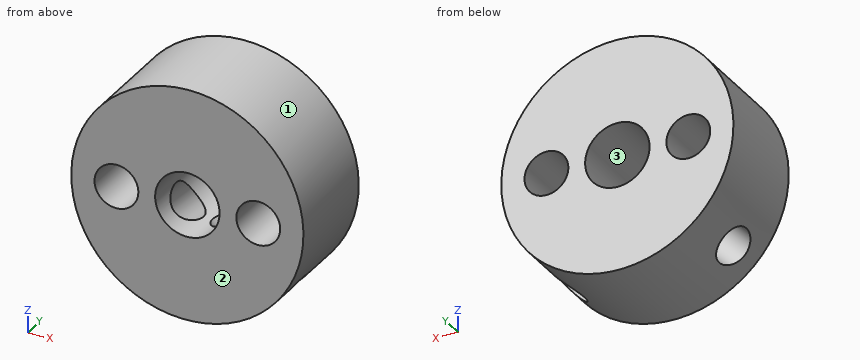
from build123d import *

# Parameters (mm, degrees)
SKETCH1_R           = 9
SKETCH1_R_2         = 2.5
SKETCH1_R_3         = 1.7
BOSS_EXTRUDE1_DEPTH = 8
SKETCH2_R           = 1.5
CUT_EXTRUDE1_DEPTH  = 16.033296378


with BuildPart() as part:
    # Sketch1 → Boss-Extrude1 (new body)
    with BuildSketch(Plane(origin=(0, 0, 0), x_dir=(1, 0, 0), z_dir=(0, 1, 0))):
        with Locations(Location((0, 0, 0), (0, 0, 270))):
            Circle(SKETCH1_R)
        with Locations(Location((0, 0, 0), (0, 0, 270))):
            Circle(SKETCH1_R_2, mode=Mode.SUBTRACT)
        with Locations(Location((5.5, 0, 0), (0, 0, 270))):
            Circle(SKETCH1_R_3, mode=Mode.SUBTRACT)
        with Locations(Location((-5.5, 0, 0), (0, 0, 90))):
            Circle(SKETCH1_R_3, mode=Mode.SUBTRACT)
    extrude(amount=BOSS_EXTRUDE1_DEPTH)

    # Sketch2 → Cut-Extrude1 (cut, through all)
    with BuildSketch(Plane(origin=(0, 0, 0), x_dir=(0, -1, 0), z_dir=(-0.7071067811865488, 0, 0.7071067811865464))):
        with Locations(Location((-3, 0, 0), (0, 0, 90))):
            Circle(SKETCH2_R)
    cut_extrude1 = extrude(amount=-CUT_EXTRUDE1_DEPTH, mode=Mode.SUBTRACT)

    # Mirror1: Cut-Extrude1 across plane
    add(cut_extrude1.mirror(Plane(origin=(0, 0, 0), x_dir=(0, 0, 1), z_dir=(1, 0, 0))), mode=Mode.SUBTRACT)


solid = part.part
Can you work these out from the model? Positions are in its coordinate system, mm. Face numbers are marked on the shaded views. Coordinates: 2 decimals unless noted, no trailing zeros. Order: outer loops, then holes, each group sorted by start corner. A loop starts at its lowest first (then second) coordinate and runs counter-clockwise, first axis right, second up. Notation, with made-up numbers: M 36.5,56.25 L 81.5,56.25 A33 ccw 81.5,91.25 Z; hole C 22.25,21.25 d4. An arc over 180 degrees is marked long. Write item = value, one per line.
(1) Suppose I cut it at A-A on x = 0. Please give me the cut outline in (y, z), plus the area to 3 significant figures.
Results are:
outline = M 0,-9 L 8,-9 L 8,-2.5 L 0,-2.5 Z; M 0,2.5 L 8,2.5 L 8,9 L 0,9 Z
area = 104 mm2
(2) For pin 1 Ø1 at (y, z) = (1, 5) entering from +X; pin 2 Ø4 at (x, z) = (0, 0) entering from -Y; pin 3 Ø2 at (x, y) = (3.5, 7) entering from -Z; pin 4 Ø2 at (y, z) = (4.5, -1.5) entering from +X, each with a flat end and sliding along its axis, tell me the tip position at first contact or that it passes through.
Results are:
pin_1 = 7.79
pin_2 = through
pin_3 = -8.65
pin_4 = 8.99
(3) Suppose I cut it at D-D on y = 5. Please give me the cut outline in (x, z), plus the area to 3 significant figures.
Results are:
outline = C 0,0 d18; hole C -5.5,0 d3.4; hole C 0,0 d5; hole C 5.5,0 d3.4
area = 217 mm2
(4) If we mould it in two halves opening along Z, with no side actions, what happens to the marked faces 1, 2 and 3? For each: pulls with the +Z half, pulls with the -Z half, needs draft (parallel to the pull), parting line crosses it, or undercut.
Results are:
face_1 = parting line crosses it
face_2 = needs draft
face_3 = undercut
(5) Suppose I cut it at C-C on z = 0. Please give me the cut outline in (x, y), plus the area to 3 significant figures.
Results are:
outline = M -9,0 L -7.2,0 L -7.2,8 L -9,8 Z; M -3.8,0 L -2.5,0 L -2.5,8 L -3.8,8 Z; M 2.5,0 L 3.8,0 L 3.8,8 L 2.5,8 Z; M 7.2,0 L 9,0 L 9,8 L 7.2,8 Z
area = 49.6 mm2
(6) I need wall thicknesses on line 1 along X through (y, z) = (5, 0); line 2 along Z through (x, y) = (4, 3.75); line 3 along Z through (x, y) = (-6, 6). Which ranges of each line are inside material? Lowest first, please. Write a range as [from, to].
Results are:
line_1 = [-9, -7.2], [-3.8, -2.5], [2.5, 3.8], [7.2, 9]
line_2 = [-8.06, -5.84], [-2.16, -0.8], [0.8, 8.06]
line_3 = [-6.71, -1.62], [1.62, 6.71]
(7) Suppose I cut it at B-B on y = 4. Please give me the cut outline in (x, z).
Results are:
outline = M -7.11,-5.52 L -2.37,-0.79 A2.5 cw long 2.37,-0.79 L 7.11,-5.52 A9 ccw long Z; M -5.52,-7.11 A9 ccw 5.52,-7.11 L 0.79,-2.37 A2.5 cw -0.79,-2.37 Z; hole C -5.5,0 d3.4; hole C 5.5,0 d3.4
